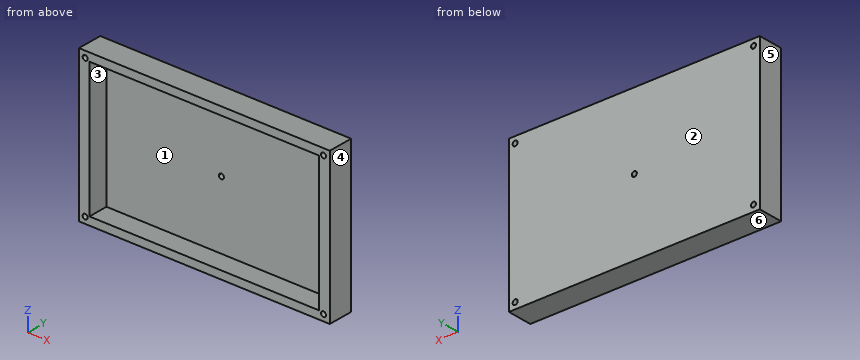
from build123d import *

# Parameters (mm, degrees)
F0_R     = 2.54
F1_DEPTH = 25.4
F2_W     = 232.68409
F2_H     = 136.17222
F3_DEPTH = 20.32


with BuildPart() as f1:
    # F0 (on Front) → F1 (new body)
    with BuildSketch(Plane.XZ):
        with BuildLine():
            Line((0, -76.2), (127, -76.2))
            Line((127, -76.2), (127, 0))
            Line((127, 0), (2.54, 0))
            ThreePointArc((2.54, 0), (1.796051, -1.796051), (0, -2.54))
            Line((0, -2.54), (0, -76.2))
        make_face()
        with Locations((120.65, -69.85)):
            Circle(F0_R, mode=Mode.SUBTRACT)
        with BuildLine():
            Line((-127, -76.2), (0, -76.2))
            Line((0, -76.2), (0, -2.54))
            ThreePointArc((0, -2.54), (-1.796051, -1.796051), (-2.54, 0))
            Line((-2.54, 0), (-127, 0))
            Line((-127, 0), (-127, -76.2))
        make_face()
        with Locations((-120.65, -69.85)):
            Circle(F0_R, mode=Mode.SUBTRACT)
        with BuildLine():
            Line((2.54, 0), (127, 0))
            Line((127, 0), (127, 76.2))
            Line((127, 76.2), (0, 76.2))
            Line((0, 76.2), (0, 2.54))
            ThreePointArc((0, 2.54), (1.796051, 1.796051), (2.54, 0))
        make_face()
        with Locations((120.65, 69.85)):
            Circle(F0_R, mode=Mode.SUBTRACT)
        with BuildLine():
            Line((-127, 69.85), (-127, 0))
            Line((-127, 0), (-2.54, 0))
            ThreePointArc((-2.54, 0), (-1.796051, 1.796051), (0, 2.54))
            Line((0, 2.54), (0, 76.2))
            Line((0, 76.2), (-120.65, 76.2))
            Line((-120.65, 76.2), (-120.65, 72.39))
            ThreePointArc((-120.65, 72.39), (-118.853949, 71.646051), (-118.11, 69.85))
            ThreePointArc((-118.11, 69.85), (-120.65, 67.31), (-123.19, 69.85))
            Line((-123.19, 69.85), (-127, 69.85))
        make_face()
        with BuildLine():
            Line((-127, 76.2), (-127, 69.85))
            Line((-127, 69.85), (-123.19, 69.85))
            ThreePointArc((-123.19, 69.85), (-122.446051, 71.646051), (-120.65, 72.39))
            Line((-120.65, 72.39), (-120.65, 76.2))
            Line((-120.65, 76.2), (-127, 76.2))
        make_face()
    extrude(amount=F1_DEPTH)

    # F2 (on face) → F3 (cut)
    with BuildSketch(Plane.XZ.offset(25.4)):
        Rectangle(F2_W, F2_H)
    extrude(amount=-F3_DEPTH, mode=Mode.SUBTRACT)


solid = f1.part
Geometry: final body of the model. Coordinates: model frame, mm. Face numbers are marked on the shaded views. A direction names the side the tool comes from. Coordinates: 2 decimals unless noted, no trailing zeros. Order: outer loops, then holes, each group sorted by start corner. A loop starts at its lowest first (then second) coordinate and runs counter-clockwise, first axis right, second up.
(1) Section query B-B (z = 33.5). Return the cut outline in (x, y), plus the area to 3 significant figures.
(2) Material intervals for probe 1 along Z at (x, y) = (120.65, -11.75); probe 2 along X at (y, z) = (-22, 64); probe 3 along Z at (x, y) = (-22, -23.5), sorted ascending.
(3) First-contact query: pin 1 (3 mm diameter, centred on x = -120.65, z = -69.85, fed in from +Y); pin 2 (12 mm diameter, centred on x = -44.5, z = 2.5, fed in from -Y). Flat tips, straight axial feed; report the tip coordinate or a pass-through.
(4) Draft query along X for the marked faces 3, 4, 5 and 6. Return one class per face: pulls with the +X half, pulls with the -X half, needs draft (parallel to the pull), parting line crosses it, or undercut.
(5) Section query C-C (x = -96). Return the cut outline in (y, z), plus the area to 3 significant figures.
(6) Section query A-A (y = -15.5). Return the cut outline in (x, z).
(7) Access query for the marked faces 1 and 2. Directions: +Z, -Z, +X, -X, +Y, -Y. A direction counts if a zero-diameter tool reaches every point of the face in a straight line with its end or side. Return the directions, or none.
Solution:
1. outline: (-127, -25.4) - (-116.34, -25.4) - (-116.34, -5.08) - (116.34, -5.08) - (116.34, -25.4) - (127, -25.4) - (127, 0) - (-127, 0) - close
1. area: 1,720 mm2
2. probe 1: z = -76.2 to -72.39, -67.31 to 67.31, 72.39 to 76.2
2. probe 2: x = -127 to -116.34, 116.34 to 127
2. probe 3: z = -76.2 to -68.09, 68.09 to 76.2
3. pin 1: passes through
3. pin 2: stops at y = -5.08
4. face 3: undercut
4. face 4: pulls with the +X half
4. face 5: pulls with the -X half
4. face 6: needs draft
5. outline: (-25.4, -76.2) - (0, -76.2) - (0, 76.2) - (-25.4, 76.2) - (-25.4, 68.09) - (-5.08, 68.09) - (-5.08, -68.09) - (-25.4, -68.09) - close
5. area: 1,100 mm2
6. outline: (-127, -76.2) - (127, -76.2) - (127, 76.2) - (-127, 76.2) - close; hole circle Ø5.08 at (-120.65, -69.85); hole circle Ø5.08 at (-120.65, 69.85); hole (-116.34, -68.09) - (116.34, -68.09) - (116.34, 68.09) - (-116.34, 68.09) - close; hole circle Ø5.08 at (120.65, -69.85); hole circle Ø5.08 at (120.65, 69.85)
7. face 1: -Y
7. face 2: +Z, -Z, +X, -X, +Y
